Read the model definition and answer for the solid it produces. Units are mm, in the model's axes. Give positions to 0.01 mm unless a question says otherwise; leave off trailing zeros. Order: outer loops, then holes, each group sorted by start corner. A loop starts at its lowest first (then second) coordinate and runs counter-clockwise, first axis right, second up.
```python
from build123d import *

# Parameters (mm, degrees)
SKETCH1_W           = 657
SKETCH1_H           = 42
BOSS_EXTRUDE1_DEPTH = 10
SKETCH2_W           = 657
SKETCH2_H           = 4
CUT_EXTRUDE1_DEPTH  = 7
SKETCH3_R           = 2
CUT_EXTRUDE2_DEPTH  = 10
CUT_EXTRUDE3_START  = -10
SKETCH4_R           = 2
CUT_EXTRUDE3_DEPTH  = 10
SKETCH5_R           = 1.5
CUT_EXTRUDE4_DEPTH  = 12


with BuildPart() as part:
    # Sketch1 → Boss-Extrude1 (new body)
    with BuildSketch(Plane.XY):
        with Locations((-281.102301223, -2.406262021)):
            Rectangle(SKETCH1_W, SKETCH1_H)
    extrude(amount=BOSS_EXTRUDE1_DEPTH)

    # Sketch2 → Cut-Extrude1 (cut)
    with BuildSketch(Plane.XY.offset(10)):
        with Locations((-281.102301223, -21.406262021)):
            Rectangle(SKETCH2_W, SKETCH2_H)
        with Locations((-281.102301223, -1.406262021)):
            Rectangle(SKETCH2_W, SKETCH2_H)
    extrude(amount=-CUT_EXTRUDE1_DEPTH, mode=Mode.SUBTRACT)

    # Sketch3 → Cut-Extrude2 (cut)
    with BuildSketch(Plane.ZY.offset(609.602301223)):
        with Locations((5, 13.593737979)):
            Circle(SKETCH3_R)
        with Locations((5, -14.406262021)):
            Circle(SKETCH3_R)
    extrude(amount=-CUT_EXTRUDE2_DEPTH, mode=Mode.SUBTRACT)

    # Sketch4 → Cut-Extrude3 (cut)
    with BuildSketch(Plane(origin=(47.397698777, 0, 0), x_dir=(0, 0, -1), z_dir=(1, 0, 0)).offset(CUT_EXTRUDE3_START)):
        with Locations(Location((-5, 13.593737979, 0), (0, 0, 180))):
            Circle(SKETCH4_R)
        with Locations(Location((-5, -14.406262021, 0), (0, 0, 180))):
            Circle(SKETCH4_R)
    extrude(amount=CUT_EXTRUDE3_DEPTH, mode=Mode.SUBTRACT)

    # Sketch5 → Cut-Extrude4 (cut)
    with BuildSketch(Plane(origin=(0, -19.406262021, 0), x_dir=(-1, 0, 0), z_dir=(0, -1, 0))):
        with Locations(Location((559.602301223, -6.5, 0), (0, 0, 90))):
            Circle(SKETCH5_R)
        with Locations(Location((281.102301223, -6.5, 0), (0, 0, 90))):
            Circle(SKETCH5_R)
        with Locations(Location((2.602301223, -6.5, 0), (0, 0, 90))):
            Circle(SKETCH5_R)
    extrude(amount=-CUT_EXTRUDE4_DEPTH, mode=Mode.SUBTRACT)


solid = part.part
```
1) The part is cut by section A-A on x = -416.5. Determine the outline of the cut face in (y, z), and give its area (3 significant figures).
Final values:
outline: (-23.41, 0) - (18.59, 0) - (18.59, 10) - (0.59, 10) - (0.59, 3) - (-3.41, 3) - (-3.41, 10) - (-19.41, 10) - (-19.41, 3) - (-23.41, 3) - close
area: 364 mm2
2) Given pin 1 (3 mm diameter, centred on y = -15, z = 5.5, fed in from -X); pin 2 (2.5 mm diameter, centred on x = -559.6, z = 6.5, fed in from -Y); pin 3 (1.2 mm diameter, centred on x = -405, y = -1, fed in from +Z); pin 4 (3.5 mm diameter, centred on x = -257, z = 7.5, fed in from -Y), each flat-ended and moving along its own axis, determine where each tip first touches the part or whether it passes through.
Final values:
pin 1: stops at x = -609.6
pin 2: stops at y = -7.41
pin 3: stops at z = 3
pin 4: stops at y = -19.41
3) Consider L1, parallel to Y at x = 44.5, z = 5; L2, parallel to X at y = -14.75, z = 6.5; L3, parallel to Y at x = -119, z = 6.25. Determine where each line is inside the solid, lowest interval first.
Final values:
L1: y = -19.41 to -16.41, -12.41 to -3.41, 0.59 to 11.59, 15.59 to 18.59
L2: x = -599.6 to -561.1, -558.1 to -282.6, -279.6 to -4.1, -1.1 to 37.4
L3: y = -19.41 to -3.41, 0.59 to 18.59
